```python
from build123d import *

# Parameters (mm, degrees)
ESBO_O1_W                = 77
ESBO_O1_H                = 135
RESSALTO_EXTRUS_O1_DEPTH = 3
ESBO_O4_W                = 3
ESBO_O4_H                = 21
CORTE_EXTRUS_O1_DEPTH    = 78.765673661
ESBO_O5_W                = 3
ESBO_O5_H                = 21
RESSALTO_EXTRUS_O2_DEPTH = 3
PADR_O_LINEAR1_COUNT     = 3
PADR_O_LINEAR1_PITCH     = 42
ESBO_O6_W                = 16
ESBO_O6_H                = 15
CORTE_EXTRUS_O2_DEPTH    = 80.293757636
PADR_O_LINEAR2_COUNT     = 2
PADR_O_LINEAR2_PITCH     = 20


with BuildPart() as part:
    # Esboço1 → Ressalto-extrusão1 (new body)
    with BuildSketch(Plane.XY):
        Rectangle(ESBO_O1_W, ESBO_O1_H)
    extrude(amount=RESSALTO_EXTRUS_O1_DEPTH)

    # Esboço4 → Corte-extrusão1 (cut, through all)
    with BuildSketch(Plane.XY.offset(3)):
        with Locations((37, 42)):
            Rectangle(ESBO_O4_W, ESBO_O4_H)
        with Locations((37, 0)):
            Rectangle(ESBO_O4_W, ESBO_O4_H)
        with Locations((37, -42)):
            Rectangle(ESBO_O4_W, ESBO_O4_H)
    extrude(amount=-CORTE_EXTRUS_O1_DEPTH, mode=Mode.SUBTRACT)

    # Esboço5 → Ressalto-extrusão2 (add)
    with BuildSketch(Plane.XY.offset(3)):
        with Locations((-40, 42)):
            Rectangle(ESBO_O5_W, ESBO_O5_H)
    ressalto_extrus_o2 = extrude(amount=-RESSALTO_EXTRUS_O2_DEPTH)

    # Padrão linear1: Ressalto-extrusão2 ×3
    with Locations(*[(0, -i * PADR_O_LINEAR1_PITCH, 0) for i in range(1, PADR_O_LINEAR1_COUNT)]):
        add(ressalto_extrus_o2)

    # Esboço6 → Corte-extrusão2 (cut, through all)
    with BuildSketch(Plane.XY.offset(3)):
        with Locations((0, -24)):
            Rectangle(ESBO_O6_W, ESBO_O6_H)
    corte_extrus_o2 = extrude(amount=-CORTE_EXTRUS_O2_DEPTH, mode=Mode.SUBTRACT)

    # Padrão linear2: Corte-extrusão2 ×2
    with Locations(*[(0, i * PADR_O_LINEAR2_PITCH, 0) for i in range(1, PADR_O_LINEAR2_COUNT)]):
        add(corte_extrus_o2, mode=Mode.SUBTRACT)


solid = part.part
```
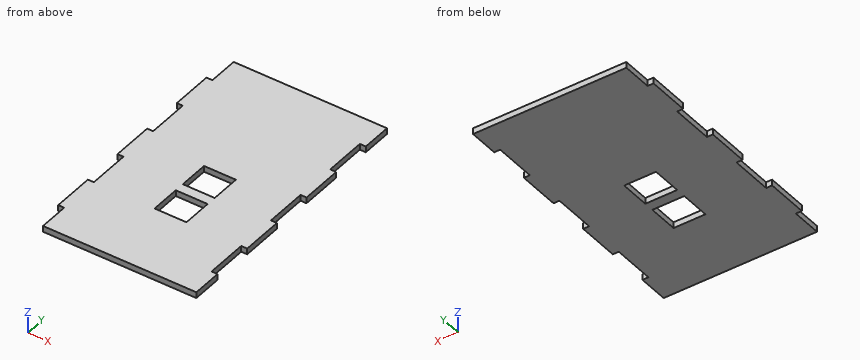
Work out the finished part from the listing and answer in its coordinate system (mm). Coordinates: 2 decimals unless noted, no trailing zeros. Loops run counter-clockwise (first coordinate to the right, second up) from the corner with the lowest first, then second, coordinate; pieces in that order, holes last. Notation, with made-up numbers: M -13,-30.75 L 9,-30.75 A27 ccw 9,5.25 Z; hole C -5,72 d1. An arc over 180 degrees is marked long. Use CSV: the item, a comma, the result in double quotes. Start each with the question number.
(1) Find section C-C, the plane y = -57.5. Give the vertices of the cut face in (x, z).
(2) Find section A-A, the plane y = 1.5. Give the vertices of the cut face in (x, z), then the cut area to 3 significant figures.
(3) Consider line 1 (X direction, y = 18, z = 1.05); line 2 (X direction, y = 42, z = 2.5). Determine where each line is inside the solid, lowest interval first.
(4) Find section B-B, the plane z = 2.35. State how many separate pieces and enclosed holes the cut face has, then the cut area to 4 significant figures.
(5) Given pin 1 Ø0.9 at (x, z) = (-40.5, 2) entering from +Y; pin 2 Ø0.9 at (x, z) = (-39.5, 1) entering from -Y; pin 3 Ø1.5 at (x, y) = (-24, 53.5) entering from -Z; pin 4 Ø1.5 at (y, z) = (-3, 1) entering from +X, each flat-ended and moving along its own axis, determine where each tip first touches the part or whether it passes through.
Recorded:
1,outline,"M -38.5,0 L 38.5,0 L 38.5,3 L -38.5,3 Z"
2,outline,"M -41.5,0 L -8,0 L -8,3 L -41.5,3 Z; M 8,0 L 35.5,0 L 35.5,3 L 8,3 Z"
2,area,"183 mm^2"
3,line 1,"x = -38.5 to 38.5"
3,line 2,"x = -41.5 to 35.5"
4,separate pieces,"1"
4,enclosed holes,"2"
4,area,"9,915 mm^2"
5,pin 1,"stops at y = 52.5"
5,pin 2,"stops at y = -52.5"
5,pin 3,"stops at z = 0"
5,pin 4,"stops at x = 35.5"
